Answer from the drawing. Dimensions are ordinates in mm from the lowest x, y and z of the part. Give positions to 0.01 mm unless a question says otherwise; leave off trailing zeros. Order: outer loops, then holes, each group sorted by start corner. A loop starts at its lowest first (then second) coordinate and runs counter-clockwise, first axis right, second up. Notation, with made-up numbers: (50.25, -16) - (84.25, -16) arc R18 ccw to (84.25, -2) - close; hole circle Ø5 at (38.5, 24.25). An arc over 180 degrees is marked (long way). Answer in a Markdown table with one row per item. Add a question column.
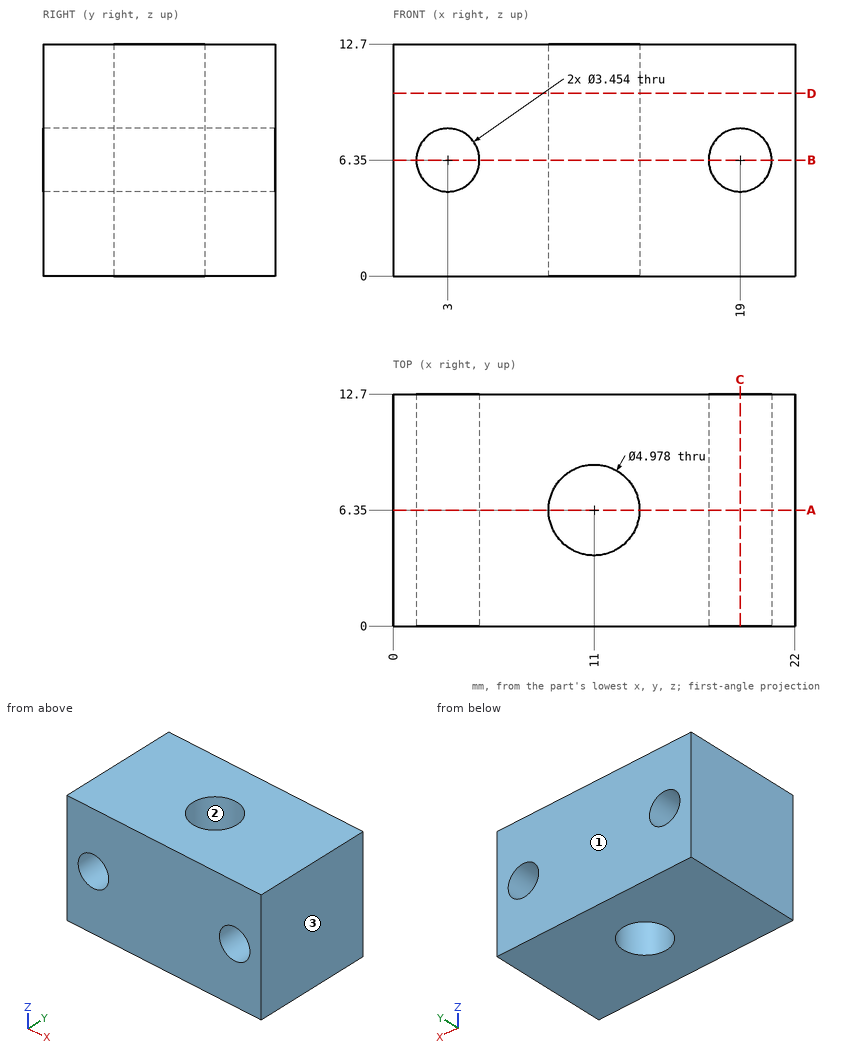
(1) Find section C-C, the plane x = 19. Write down the section's boundary in (y, z), plus the area to 3 significant figures.
(2) Straight lines are drawn through the part: line 1 (X direction, y = 6.5, z = 6.35) (1 decimal); line 2 (Y direction, x = 11, z = 8.5); line 3 (X direction, y = 10.5, z = 5) (1 decimal). For each, find the intervals that lie inside material, in ascending order.
(3) The mould has two halves that part along X. Classify the marked faces 1, 2 and 3: +X half, -X half, draft (parallel to the pull), parting line (faces both ways), or undercut.
(4) Find section B-B, the plane z = 6.35. Write down the section's boundary in (x, y).
(5) Find section A-A, the plane y = 6.35. Give the number of separate pieces and of enclosed holes in the cut face.
(6) Find section D-D, the plane z = 10. Write down the section's boundary in (x, y).
(7) This flat-tipped pin is pushed along its axis until it touches: P1, Ø3, axis at x = 19, z = 6.35, coming from the +Y side. Where does it stop, or does it pass through?
Answer key:
| question | item | result |
|---|---|---|
| 1 | outline | (0, 0) - (12.7, 0) - (12.7, 4.62) - (0, 4.62) - close; (0, 8.08) - (12.7, 8.08) - (12.7, 12.7) - (0, 12.7) - close |
| 1 | area | 117 mm² |
| 2 | line 1 | 0 to 1.3, 4.7 to 8.5, 13.5 to 17.3, 20.7 to 22 |
| 2 | line 2 | 0 to 3.86, 8.84 to 12.7 |
| 2 | line 3 | 0 to 1.9, 4.1 to 17.9, 20.1 to 22 |
| 3 | face 1 | draft |
| 3 | face 2 | undercut |
| 3 | face 3 | +X half |
| 4 | outline | (0, 0) - (1.27, 0) - (1.27, 12.7) - (0, 12.7) - close; (4.73, 0) - (17.27, 0) - (17.27, 12.7) - (4.73, 12.7) - close; (20.73, 0) - (22, 0) - (22, 12.7) - (20.73, 12.7) - close; hole circle Ø4.98 at (11, 6.35) |
| 5 | separate pieces | 2 |
| 5 | enclosed holes | 2 |
| 6 | outline | (0, 0) - (22, 0) - (22, 12.7) - (0, 12.7) - close; hole circle Ø4.98 at (11, 6.35) |
| 7 | P1 | through |
